Autodesk Inventor part; units mm, degrees
ref_plane "YZ Plane" through (0, 0, 0) normal (1, 0, 0) x (0, 1, 0)
ref_plane "XZ Plane" through (0, 0, 0) normal (0, 1, 0) x (-1, 0, 0)
ref_plane "XY Plane" through (0, 0, 0) normal (0, 0, 1) x (1, 0, 0)
sketch "Sketch1" plane through (0, 0, 0) normal (0, 1, 0) x (-1, 0, 0)
  line L0 (0, 0) -> (-25.4, 0)
  line L1 (-25.4, 0) -> (-25.4, -45.72)
  line L2 (0, -76.2) -> (0, 0)
  line L3 (-25.4, 0) -> (-25.4, -45.72)
  line L4 (-25.4, -45.72) -> (0, -76.2)
  point P0 (0, -76.2)
  dimension "d2" = 45.72
  dimension "d22" = 25.4
  dimension "d23" = 76.2
extrude "Extrusion1" add sketch "Sketch1" along normal blind 5.08
fillet "Fillet2" radius 12.7 1 edges at (25.4, 2.54, 0)
fillet "Fillet3" radius 12.7 1 edges at (0, 2.54, 0)
sketch "Sketch2" plane through (0, 5.08, 0) normal (0, 1, 0) x (1, 0, 0)
  circle A0 centre (12.7, 12.7) radius 3.175
  circle A1 centre (12.7, 50.8) radius 3.175
  point P0 (0, 0)
  dimension "d9" = 6.35
  dimension "d10" = 12.7
  dimension "d11" = 12.7
  dimension "d16" = 6.35
  dimension "d17" = 38.1
  dimension "d18" = 12.7
extrude "Extrusion2" cut sketch "Sketch2" against normal blind 12.7
fillet "Fillet6" radius 3.175 1 edges at (0, 2.54, -76.2)
properties part number "Finger"
Input: part model. Units: mm. Frame: model coordinates. Give positions to 0.01 mm unless a question says otherwise; leave off trailing zeros. Order: outer loops, then holes, each group sorted by start corner. A loop starts at its lowest first (then second) coordinate and runs counter-clockwise, first axis right, second up. Notation, with made-up numbers: M 5.25,3.5 L 21.25,3.5 A17 ccw 21.25,12.5 Z; hole C -35.5,19.5 d10. An arc over 180 degrees is marked long. Return JSON: item names as keys, results as strings.
Item 1: Cut plane A-A (y = 3.3). State how many separate pieces and enclosed holes the cut face has, then the cut area to 3 significant figures.
Solutions:
{"separate pieces": "1", "enclosed holes": "2", "area": "1,400 mm^2"}
Item 2: Cut plane C-C (z = -10.5). Return loops of the section in (x, y).
Solutions:
{"outline": "M 0.19,0 L 10.41,0 L 10.41,5.08 L 0.19,5.08 Z; M 14.99,0 L 25.21,0 L 25.21,5.08 L 14.99,5.08 Z"}
Item 3: Cut plane B-B (z = -50.8). Return loops of the section in (x, y) (3 decimals).
Solutions:
{"outline": "M 0,0 L 9.525,0 L 9.525,5.08 L 0,5.08 Z; M 15.875,0 L 21.167,0 L 21.167,5.08 L 15.875,5.08 Z"}
Item 4: First-contact query: P1, Ø2, axis at x = 6.5, y = 3.5, coming from the +Z side; P2, Ø1, axis at x = 21.5, y = 4, coming from the +Z side; P3, Ø5, axis at x = 12.7, z = -12.7, coming from the -Y side. Flat tips, straight axial feed; report the tip coordinate or a pass-through.
Solutions:
{"P1": "z = -1.11", "P2": "z = -3.09", "P3": "through"}
Item 5: Pull-direction query (X, two-part tool) for faces 1 (the cylindrical face through (2.145, 2.576, -70.434)), 2 (the flat face through (25.4, 3, -29)), 3 (the cylindrical face through (10.18, 2.58, -10.77)), 4 (the cylindrical face through (12.29, 2.58, -53.95)); classes: +X half, -X half, draft (parallel to the pull), parting line (faces both ways), or undercut.
Solutions:
{"face 1": "parting line", "face 2": "+X half", "face 3": "undercut", "face 4": "undercut"}
Item 6: Ray query, probe 1 along X at (y, z) = (1.9, -12.7) (3 decimals); probe 2 along Z at (x, y) = (12.7, 3.9) (3 decimals); probe 3 along Z at (x, y) = (13, 0.35). Return the intervals inside material, ascending.
Solutions:
{"probe 1": "0 to 9.525, 15.875 to 25.4", "probe 2": "-60.96 to -53.975, -47.625 to -15.875, -9.525 to 0", "probe 3": "-60.6 to -53.96, -47.64 to -15.86, -9.54 to 0"}
Item 7: Cut plane D-D (x = 6.75). Return loops of the section in (y, z), then the cut area to 3 significant figures.
Solutions:
{"outline": "M 0,-68.1 L 5.08,-68.1 L 5.08,-1.48 L 0,-1.48 Z", "area": "338 mm^2"}
